```python
from build123d import *

# Parameters (mm, degrees)
SKETCH1_W                 = 70.4
SKETCH1_H                 = 2
BOSS_EXTRUDE2_DEPTH       = 10
SKETCH2_W                 = 2
SKETCH2_H                 = 55
BOSS_EXTRUDE3_DEPTH       = 10
SKETCH3_W                 = 19
SKETCH3_H                 = 3
BOSS_EXTRUDE4_DEPTH       = 2
SKETCH4_W                 = 15
SKETCH4_H                 = 10
CUT_EXTRUDE2_DEPTH        = 2
SKETCH5_W                 = 2
SKETCH5_H                 = 3
BOSS_EXTRUDE5_DEPTH       = 1
SKETCH6_W                 = 2
SKETCH6_H                 = 3
BOSS_EXTRUDE6_DEPTH       = 1
SKETCH7_W                 = 57
SKETCH7_H                 = 2
BOSS_EXTRUDE7_DEPTH       = 6.6
SKETCH8_W                 = 57
SKETCH8_H                 = 2
BOSS_EXTRUDE8_DEPTH       = 6.6
BOSS_EXTRUDE9_DEPTH       = 5
SKETCH12_W                = 2
SKETCH12_H                = 5
SKETCH12_H_2              = 40
SKETCH12_H_3              = 30
BOSS_EXTRUDE10_DEPTH      = 20
BOSS_EXTRUDE11_DEPTH      = 3
SKETCH14_W                = 0.5
SKETCH14_H                = 9
CUT_EXTRUDE3_DEPTH        = 3
SKETCH15_W                = 38.4
SKETCH15_H                = 45
CUT_EXTRUDE4_DEPTH        = 3
BOSS_EXTRUDE12_DEPTH      = 0.5
SKETCH17_R                = 1.8
SKETCH17_W                = 3
SKETCH17_H                = 5
CUT_EXTRUDE6_DEPTH        = 3
CUT_EXTRUDE7_DEPTH        = 116
CUT_EXTRUDE7_DEPTH_BACK   = 44
SKETCH18_W                = 45
SKETCH18_H                = 3
SKETCH19_R                = 1.8
CUT_EXTRUDE8_DEPTH        = 10
SKETCH20_R                = 1.8
CUT_EXTRUDE9_DEPTH        = 10
BOSS_EXTRUDE15_DEPTH      = 2
BOSS_EXTRUDE15_DEPTH_BACK = 23
SKETCH25_W                = 2.5
SKETCH25_H                = 4


with BuildPart() as part:
    # Sketch1 → Boss-Extrude2 (new body)
    with BuildSketch(Plane(origin=(0, 0, 0), x_dir=(1, 0, 0), z_dir=(0, 1, 0))):
        with Locations((35.2, 1)):
            Rectangle(SKETCH1_W, SKETCH1_H)
    extrude(amount=BOSS_EXTRUDE2_DEPTH)

    # Sketch2 → Boss-Extrude3 (add)
    with BuildSketch(Plane(origin=(0, 10, 0), x_dir=(1, 0, 0), z_dir=(0, 1, 0))):
        with Locations((1, 29.5)):
            Rectangle(SKETCH2_W, SKETCH2_H)
        with Locations((69.4, 29.5)):
            Rectangle(SKETCH2_W, SKETCH2_H)
    extrude(amount=-BOSS_EXTRUDE3_DEPTH)

    # Sketch3 → Boss-Extrude4 (add)
    with BuildSketch(Plane.XY):
        with Locations((35.2, 11.5)):
            Rectangle(SKETCH3_W, SKETCH3_H)
    extrude(amount=-BOSS_EXTRUDE4_DEPTH)

    # Sketch4 → Cut-Extrude2 (cut)
    with BuildSketch(Plane.XY):
        with Locations((35.2, 5)):
            Rectangle(SKETCH4_W, SKETCH4_H)
    extrude(amount=-CUT_EXTRUDE2_DEPTH, mode=Mode.SUBTRACT)

    # Sketch5 → Boss-Extrude5 (add)
    with BuildSketch(Plane.ZY.offset(-25.7)):
        with Locations((-1, 11.5)):
            Rectangle(SKETCH5_W, SKETCH5_H)
    extrude(amount=BOSS_EXTRUDE5_DEPTH)

    # Sketch6 → Boss-Extrude6 (add)
    with BuildSketch(Plane(origin=(44.7, 0, 0), x_dir=(0, 0, -1), z_dir=(1, 0, 0))):
        with Locations((1, 11.5)):
            Rectangle(SKETCH6_W, SKETCH6_H)
    extrude(amount=BOSS_EXTRUDE6_DEPTH)

    # Sketch7 → Boss-Extrude7 (add)
    with BuildSketch(Plane.ZY):
        with Locations((-28.5, 1)):
            Rectangle(SKETCH7_W, SKETCH7_H)
    extrude(amount=BOSS_EXTRUDE7_DEPTH)

    # Sketch8 → Boss-Extrude8 (add)
    with BuildSketch(Plane(origin=(70.4, 0, 0), x_dir=(0, 0, -1), z_dir=(1, 0, 0))):
        with Locations((28.5, 1)):
            Rectangle(SKETCH8_W, SKETCH8_H)
    extrude(amount=BOSS_EXTRUDE8_DEPTH)

    # Sketch10 → Boss-Extrude9 (add)
    with BuildSketch(Plane(origin=(0, 0, -57), x_dir=(-1, 0, 0), z_dir=(0, 0, -1))):
        Polygon((-2, 10), (-2, 0), (6.6, 0), (6.6, 2), (0, 2), (0, 10), align=None)
        Polygon((-77, 0), (-68.4, 0), (-68.4, 10), (-70.4, 10), (-70.4, 2), (-77, 2), align=None)
    extrude(amount=BOSS_EXTRUDE9_DEPTH)

    # Sketch12 → Boss-Extrude10 (add)
    with BuildSketch(Plane(origin=(0, 10, 0), x_dir=(1, 0, 0), z_dir=(0, 1, 0))):
        with Locations((1, 59.5)):
            Rectangle(SKETCH12_W, SKETCH12_H)
        with Locations((1, 37)):
            Rectangle(SKETCH12_W, SKETCH12_H_2)
        with Locations((69.4, 42)):
            Rectangle(SKETCH12_W, SKETCH12_H_3)
        with Locations((69.4, 59.5)):
            Rectangle(SKETCH12_W, SKETCH12_H)
    extrude(amount=BOSS_EXTRUDE10_DEPTH)

    # Sketch13 → Boss-Extrude11 (add)
    with BuildSketch(Plane(origin=(0, 30, 0), x_dir=(1, 0, 0), z_dir=(0, 1, 0))):
        Polygon((0, 17), (35.2, 17), (35.2, 27), (70.4, 27), (70.4, 62), (0, 62), align=None)
    extrude(amount=BOSS_EXTRUDE11_DEPTH)

    # Sketch14 → Cut-Extrude3 (cut)
    with BuildSketch(Plane(origin=(0, 33, 0), x_dir=(1, 0, 0), z_dir=(0, 1, 0))):
        with Locations((11.7, 51)):
            Rectangle(SKETCH14_W, SKETCH14_H)
        with Locations((11.7, 38)):
            Rectangle(SKETCH14_W, SKETCH14_H)
        with Locations((11.7, 25.5)):
            Rectangle(SKETCH14_W, SKETCH14_H)
        with Locations((58.2, 51)):
            Rectangle(SKETCH14_W, SKETCH14_H)
        with Locations((58.2, 38)):
            Rectangle(SKETCH14_W, SKETCH14_H)
    extrude(amount=-CUT_EXTRUDE3_DEPTH, mode=Mode.SUBTRACT)

    # Sketch15 → Cut-Extrude4 (cut)
    with BuildSketch(Plane(origin=(0, 33, 0), x_dir=(1, 0, 0), z_dir=(0, 1, 0))):
        with Locations((35.2, 39.5)):
            Rectangle(SKETCH15_W, SKETCH15_H)
    extrude(amount=-CUT_EXTRUDE4_DEPTH, mode=Mode.SUBTRACT)

    # Sketch16 → Boss-Extrude12 (add)
    with BuildSketch(Plane.XY):
        Polygon((-6.6, 0), (27.7, 0), (27.7, 10), (42.7, 10), (42.7, 0), (77, 0), (77, 2), (70.4, 2), (70.4, 10), (45.7, 10), (45.7, 13), (24.7, 13), (24.7, 10), (0, 10), (0, 2), (-6.6, 2), align=None)
    extrude(amount=BOSS_EXTRUDE12_DEPTH)

    # Sketch17 → Cut-Extrude6 (cut)
    with BuildSketch(Plane(origin=(0, 2, 0), x_dir=(1, 0, 0), z_dir=(0, 1, 0))):
        with Locations(Location((-3.3, 55, 0), (0, 0, 270))):
            Circle(SKETCH17_R)
        with Locations(Location((73.7, 55, 0), (0, 0, 270))):
            Circle(SKETCH17_R)
        with Locations(Location((-3.3, 6.5, 0), (0, 0, 270))):
            Circle(SKETCH17_R)
        with Locations(Location((73.7, 6.5, 0), (0, 0, 270))):
            Circle(SKETCH17_R)
        with Locations(Location((-3.3, 30.75, 0), (0, 0, 270))):
            Circle(SKETCH17_R)
        with Locations(Location((73.7, 30.75, 0), (0, 0, 270))):
            Circle(SKETCH17_R)
        with Locations((-3.3, 14.5)):
            Rectangle(SKETCH17_W, SKETCH17_H)
        with Locations((73.7, 14.5)):
            Rectangle(SKETCH17_W, SKETCH17_H)
    extrude(amount=-CUT_EXTRUDE6_DEPTH, mode=Mode.SUBTRACT)

    # Sketch18 → Cut-Extrude7 (cut, two sides: drawn at the far end of the back side and taken through both)
    with BuildSketch(Plane(origin=(16, 0, 0), x_dir=(0, 0, -1), z_dir=(1, 0, 0)).offset(-CUT_EXTRUDE7_DEPTH_BACK)):
        with Locations((39.5, 31.5)):
            Rectangle(SKETCH18_W, SKETCH18_H)
    extrude(amount=CUT_EXTRUDE7_DEPTH + CUT_EXTRUDE7_DEPTH_BACK, mode=Mode.SUBTRACT)

    # Sketch19 → Cut-Extrude8 (cut)
    with BuildSketch(Plane(origin=(2, 0, 0), x_dir=(0, 0, -1), z_dir=(1, 0, 0))):
        with Locations((52, 26)):
            Circle(SKETCH19_R)
        with Locations((27, 26)):
            Circle(SKETCH19_R)
    extrude(amount=-CUT_EXTRUDE8_DEPTH, mode=Mode.SUBTRACT)

    # Sketch20 → Cut-Extrude9 (cut)
    with BuildSketch(Plane(origin=(70.4, 0, 0), x_dir=(0, 0, -1), z_dir=(1, 0, 0))):
        with Locations((52, 26)):
            Circle(SKETCH20_R)
        with Locations((37, 26)):
            Circle(SKETCH20_R)
    extrude(amount=-CUT_EXTRUDE9_DEPTH, mode=Mode.SUBTRACT)

    # Sketch25 → Boss-Extrude15 (add, two sides: drawn at the far end of the back side and taken through both)
    with BuildSketch(Plane.ZY.offset(-24.7).offset(-BOSS_EXTRUDE15_DEPTH_BACK)):
        with Locations((-0.75, 12)):
            Rectangle(SKETCH25_W, SKETCH25_H)
    extrude(amount=BOSS_EXTRUDE15_DEPTH + BOSS_EXTRUDE15_DEPTH_BACK)


solid = part.part
```
Build history of the part. All positions in model axes, mm. A direction names the side the tool comes from. Round coordinates to 2 decimals unless told otherwise and drop trailing zeros. Loops run counter-clockwise (first coordinate to the right, second up) from the corner with the lowest first, then second, coordinate; pieces in that order, holes last.
Item 1: Pin check, flat tips, straight feed: P1, Ø2, axis at y = 26, z = -52, coming from the -X side; P2, Ø2, axis at x = 64, y = 8, coming from the -Z side; P3, Ø6, axis at x = -3.3, z = -55, coming from the +Y side; P4, Ø1, axis at x = 1, y = 24.5, coming from the +Z side. Stop position of each tip, or through.
Item 2: Which spindle directions (+Z, -Z, +X, -X, +Y, -Y) get a long thin tool onto all of the face, cutting with end or side? Do faces 4 (the face through (-1, 2, -31)), 5 (the face through (35, 10, -1)), 6 (the face through (69, 10, -7)), 7 (the face through (72.2, 1, -14)), 8 (the face through (76, 2, -31)). Say none if no direction does.
Item 3: Saw through at A-A (z = -6.5). List the corners of the cut face in (x, y), then the cut area to 3 significant figures.
Item 4: Saw through at C-C (z = -45). List the corners of the cut face in (x, y), then the cut area to 3 significant figures.
Item 5: Saw through at D-D (x = 73.7). List the corners of the cut face in (y, z).
Item 6: Two-plate mould, pull along Z, no slides. Class faces 1 (the face through (-1.8, 1, -14)), 2 (the face through (69, 20, -27)), 3 (the face through (-6.6, 1, -31)): released by +Z, released by -Z, zero draft, split by the parting line, or undercut.
Item 7: Drill centre lines: line 1 along X through (y, z) = (0.6, -6.5); line 2 along Z through (x, y) = (73.7, 1.2); line 3 along X through (y, z) = (18, -50.5). Where is each one in solid material? Low to high.
Item 8: Saw through at B-B (y = 15). List the corners of the cut face in (x, z), then the cut area to 3 significant figures.
Worked answers:
1. P1: passes through
1. P2: stops at z = -2
1. P3: stops at y = 2
1. P4: stops at z = -17
2. face 4: +Z, -Z, -X, +Y
2. face 5: +Z, -Z, -Y
2. face 6: +Z, +X, +Y
2. face 7: +Y, -Y
2. face 8: +Z, -Z, +X, +Y
3. outline: (-6.6, 0) - (-5.1, 0) - (-5.1, 2) - (-6.6, 2) - close; (-1.5, 0) - (2, 0) - (2, 10) - (0, 10) - (0, 2) - (-1.5, 2) - close; (68.4, 0) - (71.9, 0) - (71.9, 2) - (70.4, 2) - (70.4, 10) - (68.4, 10) - close; (75.5, 0) - (77, 0) - (77, 2) - (75.5, 2) - close
3. area: 52.0 mm2
4. outline: (-6.6, 0) - (2, 0) - (2, 30) - (0, 30) - (0, 2) - (-6.6, 2) - close; (68.4, 0) - (77, 0) - (77, 2) - (70.4, 2) - (70.4, 30) - (68.4, 30) - close
4. area: 146 mm2
5. outline: (0, -62) - (2, -62) - (2, -56.8) - (0, -56.8) - close; (0, -53.2) - (2, -53.2) - (2, -32.55) - (0, -32.55) - close; (0, -28.95) - (2, -28.95) - (2, -17) - (0, -17) - close; (0, -12) - (2, -12) - (2, -8.3) - (0, -8.3) - close; (0, -4.7) - (2, -4.7) - (2, 0.5) - (0, 0.5) - close
6. face 1: undercut
6. face 2: released by +Z
6. face 3: zero draft
7. line 1: x = -6.6 to -5.1, -1.5 to 2, 68.4 to 71.9, 75.5 to 77
7. line 2: z = -62 to -56.8, -53.2 to -32.55, -28.95 to -17, -12 to -8.3, -4.7 to 0.5
7. line 3: x = 0 to 2, 68.4 to 70.4
8. outline: (0, -62) - (2, -62) - (2, -17) - (0, -17) - close; (68.4, -62) - (70.4, -62) - (70.4, -27) - (68.4, -27) - close
8. area: 160 mm2
